Design review of the part built by this model. Coordinates are the model's own, in mm. Face numbers are marked on the shaded views. Coordinates: 2 decimals unless noted, no trailing zeros. Loops run counter-clockwise (first coordinate to the right, second up) from the corner with the lowest first, then second, coordinate; pieces in that order, holes last. Notation, with made-up numbers: (-12, 70) -> (1, 70) arc R29 cw to (1, 96) -> close; hole circle Ø6 at (8.5, -32). An arc over 180 degrees is marked (long way). Answer in a Markdown table with one row per item.
```python
from build123d import *

# Parameters (mm, degrees)
SKETCH_1_R      = 5.25
SKETCH_1_R_2    = 3.5
EXTRUDE_1_DEPTH = 4
FILLET_1_R      = 0.5


with BuildPart() as part:
    # 草图1 → 凸台-拉伸1 (new body)
    with BuildSketch(Plane(origin=(0, 0, 0), x_dir=(1, 0, 0), z_dir=(0, 1, 0))):
        with BuildLine():
            ThreePointArc((2.725960977, 8.577245289), (-9, 0), (2.725960977, -8.577245289))
            ThreePointArc((2.725960977, -8.577245289), (25.580430084, -4.227861915), (48.814522163, -5.419859889))
            ThreePointArc((48.814522163, -5.419859889), (55.25, 0), (48.814522163, 5.419859889))
            ThreePointArc((48.814522163, 5.419859889), (25.580430084, 4.227861915), (2.725960977, 8.577245289))
        make_face()
        with Locations(Location((0, 0, 0), (0, 0, 270))):
            Circle(SKETCH_1_R, mode=Mode.SUBTRACT)
        with Locations(Location((49.75, 0, 0), (0, 0, 270))):
            Circle(SKETCH_1_R_2, mode=Mode.SUBTRACT)
    extrude(amount=EXTRUDE_1_DEPTH)

    # 圆角1
    fillet_1_edges = [part.edges().sort_by_distance(p)[0] for p in [
        (25.580430084, 4, 4.227861915),
        (55.25, 4, 0),
        (25.580430084, 4, -4.227861915),
        (55.25, 0, 0),
        (25.580430084, 0, 4.227861915),
        (-9, 0, 0),
        (25.580430084, 0, -4.227861915),
        (-9, 4, 0),
    ]]
    fillet(fillet_1_edges, radius=FILLET_1_R)


solid = part.part
```
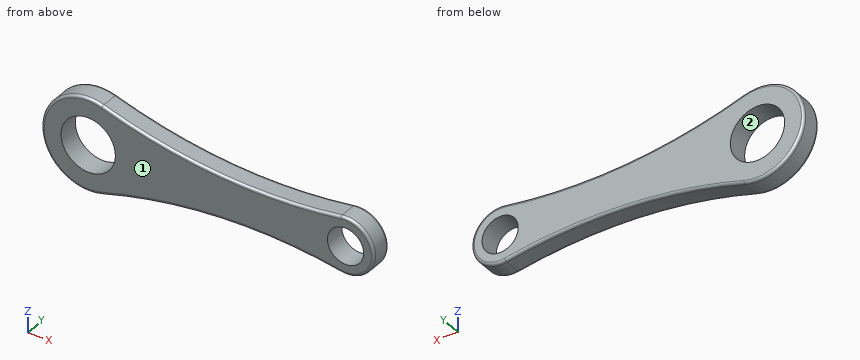
(1) Take a section at B-B on y = 2.05. Give the boundary of the cut face in (x, z).
Evaluation:
| item | result |
|---|---|
| outline | (2.73, -8.58) arc R97.44 cw to (48.81, -5.42) arc R5.5 ccw (long way) to (48.81, 5.42) arc R97.44 cw to (2.73, 8.58) arc R9 ccw (long way) to start; hole circle Ø10.5 at (0, 0); hole circle Ø7 at (49.75, 0) |
(2) For pin 1 (6 mm diameter, centred on x = 47.5, z = 4.5, fed in from -Y); pin 2 (1.5 mm diameter, centred on x = 24.5, y = 1, fed in from -Z), all flat-tipped, find the tip position at first contact; note any pin that passes through.
Evaluation:
| item | result |
|---|---|
| pin 1 | stops at y = 0 |
| pin 2 | stops at z = -4.37 |
(3) To check wall thickness, follow probe 1 along X at (y, z) = (2.95, 0); probe 2 along X at (y, z) = (1.4, -2.5); probe 3 along Z at (x, y) = (4, 0.25). State the ranges of each line that lie inside material, in increasing order.
Evaluation:
| item | result |
|---|---|
| probe 1 | x = -9 to -5.25, 5.25 to 46.25, 53.25 to 55.25 |
| probe 2 | x = -8.65 to -4.62, 4.62 to 47.3, 52.2 to 54.65 |
| probe 3 | z = -8.11 to -3.4, 3.4 to 8.11 |
(4) Draft analysis for pull direction Z (two halves, no side actions). For the marked faces 1 and 2, state which applies: pulls with the +Z half, pulls with the -Z half, needs draft (parallel to the pull), parting line crosses it, or undercut.
Evaluation:
| item | result |
|---|---|
| face 1 | needs draft |
| face 2 | undercut |
(5) Take a section at A-A on z = 0. Give the boundary of the cut face in (x, y).
Evaluation:
| item | result |
|---|---|
| outline | (-9, 0.5) arc R0.5 ccw to (-8.5, 0) -> (-5.25, 0) -> (-5.25, 4) -> (-8.5, 4) arc R0.5 ccw to (-9, 3.5) -> close; (5.25, 0) -> (46.25, 0) -> (46.25, 4) -> (5.25, 4) -> close; (53.25, 0) -> (54.75, 0) arc R0.5 ccw to (55.25, 0.5) -> (55.25, 3.5) arc R0.5 ccw to (54.75, 4) -> (53.25, 4) -> close |
